For this review, take the finished solid that the model builds, in its own axes (mm). A direction names the side the tool comes from. Give positions to 0.01 mm unless a question says otherwise; leave off trailing zeros. Write each loop counter-clockwise with the first axis right and the second up, starting at its lowest first coordinate (ties: lowest second). Pieces come first, ordered by that corner, then holes.
Q1. We need section A-A (z = 15.5). Write out the cut boundary in (x, y), then the cut area to 3 significant figures.
Q2. Insertion check: P1, Ø10, axis at x = -17, z = 13, coming from the +Y side; P2, Ø4, axis at x = -7, z = 0.5, coming from the -Y side; P3, Ø1.5, axis at x = -12.5, z = 25, coming from the +Y side. Each pin has a flat end and moves straight along its axis. Give the tip position at first contact, or say it passes through.
Q3. For line 1 (Y direction, x = 0, z = 23); line 2 (Y direction, x = 0, z = 38); line 3 (Z direction, x = 7, y = -8), list the stretches that pass through material, from the lowest coordinate up.
Q4. We need section C-C (x = 10.5). Write out the cut boundary in (y, z), then the cut area to 3 significant figures.
Q5. Machinability: for faces 1 (the flat face through (-11, 17, 10)), 2 (the flat face through (3, 15, 42.7)), which of the approach directions +Z, -Z, +X, -X, +Y, -Y give a long, thin tool a straight path to every point of the face, cutting with its end or side? Answer none if there is none.
Q6. Mouldability with a two-part tool opening along X and no side actions: class faces 3 (the cylindrical face through (-4.336, 19.524, 26.121)), 4 (the cylindrical face through (-0.867, -3.905, 19.988)), 5 (the flat face through (0, 0, -10)), 6 (the conical face through (0, 1, 7)) as released by +X, released by -X, zero draft, split by the parting line, or undercut.
Q7. We need section D-D (z = -2.5). Write out the cut boundary in (x, y), then the cut area to 3 significant figures.
Q8. We need section B-B (y = 6). Write out the cut boundary in (x, z).
Solid Edge part; units mm, degrees
sketch "Sketch1" plane through (0, 0, 0) normal (0, 0, 1) x (1, 0, 0)
  circle A0 centre (0, 0) radius 25
extrude "Protrusion1" add sketch "Sketch1" along normal blind 10
sketch "Sketch2" plane through (0, 0, 0) normal (1, 0, 0) x (0, 1, 0)
  line L0 (0, 10) -> (4, 10)
  line L1 (4, 10) -> (0, 6)
  line L2 (0, 10) -> (0, 6)
revolve "RevolvedCutout1" cut sketch "Sketch2" angle 360 about axis through (0, 0, 0) along (0, 0, 1)
sketch "Sketch3" plane through (0, 0, 10) normal (0, 0, 1) x (1, 0, 0)
  circle A0 centre (0, 0) radius 20
extrude "Protrusion2" add sketch "Sketch3" along normal blind 32.7
sketch "Sketch4" plane through (0, 0, 42.7) normal (0, 0, 1) x (1, 0, 0)
  circle A0 centre (0, 0) radius 15
extrude "ExtrudedCutout_2" cut sketch "Sketch4" against normal blind 12
sketch "Sketch5" plane through (0, 0, 30.7) normal (0, 0, 1) x (1, 0, 0)
  circle A0 centre (0, 0) radius 4
extrude "ExtrudedCutout_3" cut sketch "Sketch5" against normal blind 20.7
cosmetic_thread "Thread1"
sketch "Sketch6" plane through (0, 0, 0) normal (0, 1, 0) x (-1, 0, 0)
  line L0 (-5, 30.7) -> (-4, 29.7)
  line L1 (-4, 29.7) -> (-4, 30.7)
  line L2 (-4, 30.7) -> (-5, 30.7)
revolve "RevolvedCutout2" cut sketch "Sketch6" angle 360 about axis through (0, 0, 0) along (0, 0, 1)
sketch "Sketch7" plane through (0, 0, 0) normal (0, 0, -1) x (-1, 0, 0)
  circle A0 centre (0, 0) radius 25
extrude "ExtrudedProtrusion_4" add sketch "Sketch7" along normal blind 10
properties material "Steel - Stainless:1.4301 , X5CrNi18-10"
Computed:
1. outline: circle Ø40 at (0, 0); hole circle Ø8 at (0, 0)
1. area: 1,210 mm2
2. P1: stops at y = 21.35
2. P2: stops at y = -24.49
2. P3: stops at y = 16.18
3. line 1: y = -20 to -4, 4 to 20
3. line 2: y = -20 to -15, 15 to 20
3. line 3: z = -10 to 30.7
4. outline: (-22.69, -10) - (22.69, -10) - (22.69, 10) - (17.02, 10) - (17.02, 42.7) - (10.71, 42.7) - (10.71, 30.7) - (-10.71, 30.7) - (-10.71, 42.7) - (-17.02, 42.7) - (-17.02, 10) - (-22.69, 10) - close
4. area: 1,760 mm2
5. face 1: +Z
5. face 2: +Z, +X, -X, +Y, -Y
6. face 3: split by the parting line
6. face 4: undercut
6. face 5: zero draft
6. face 6: undercut
7. outline: circle Ø50 at (0, 0)
7. area: 1,960 mm2
8. outline: (-24.27, -10) - (24.27, -10) - (24.27, 10) - (19.08, 10) - (19.08, 42.7) - (13.75, 42.7) - (13.75, 30.7) - (-13.75, 30.7) - (-13.75, 42.7) - (-19.08, 42.7) - (-19.08, 10) - (-24.27, 10) - close
